Part model, mm, in its own coordinate system. A direction names the side the tool comes from. Give positions to 0.01 mm unless a question says otherwise; leave off trailing zeros. Loops run counter-clockwise (first coordinate to the right, second up) from the corner with the lowest first, then second, coordinate; pieces in that order, holes last. Notation, with made-up numbers: (21, -25) -> (75, -25) arc R8 ccw to (75, -16) -> close; hole circle Ø6 at (-8.5, 49.25). An arc over 180 degrees is marked (long way). Write item = value, one per line.
from build123d import *

# Parameters (mm, degrees)
SKETCH_1_W          = 12.5
SKETCH_1_H          = 12.5
EXTRUDE_1_DEPTH     = 44.8
SKETCH_2_W          = 10
SKETCH_2_H          = 10
CUT_EXTRUDE_1_DEPTH = 44
FILLET_1_R          = 1


with BuildPart() as part:
    # Эскиз1 → Бобышка-Вытянуть1 (new body)
    with BuildSketch(Plane(origin=(0, 0, 0), x_dir=(1, 0, 0), z_dir=(0, 1, 0))):
        with Locations((6.25, 6.25)):
            Rectangle(SKETCH_1_W, SKETCH_1_H)
    extrude(amount=EXTRUDE_1_DEPTH)

    # Эскиз2 → Вырез-Вытянуть1 (cut)
    with BuildSketch(Plane(origin=(0, 44.8, 0), x_dir=(1, 0, 0), z_dir=(0, 1, 0))):
        with Locations((6.25, 6.25)):
            Rectangle(SKETCH_2_W, SKETCH_2_H)
    extrude(amount=-CUT_EXTRUDE_1_DEPTH, mode=Mode.SUBTRACT)

    # Скругление1
    fillet_1_edges = [part.edges().sort_by_distance(p)[0] for p in [
        (6.25, 0, -12.5),
        (6.25, 0, 0),
    ]]
    fillet(fillet_1_edges, radius=FILLET_1_R)


solid = part.part
1) Slice it at B-B, the plane x = 4.75. List the corners of the cut face in (y, z), and give its area (3 significant figures).
Resolved:
outline = (0, -11.5) arc R1 ccw to (1, -12.5) -> (44.8, -12.5) -> (44.8, -11.25) -> (0.8, -11.25) -> (0.8, -1.25) -> (44.8, -1.25) -> (44.8, 0) -> (1, 0) arc R1 ccw to (0, -1) -> close
area = 120 mm²
2) Drill centre lines: line 1 along Z through (x, y) = (11, 18.5); line 2 along X through (y, z) = (7, -8.5); line 3 along Y through (x, z) = (4.75, -10). Where is each one in solid material? Low to high. Write a range as [from, to].
Resolved:
line_1 = [-12.5, -11.25], [-1.25, 0]
line_2 = [0, 1.25], [11.25, 12.5]
line_3 = [0, 0.8]
3) Slice it at C-C, the plane y = 19.5. List the corners of the cut face in (x, z).
Resolved:
outline = (0, -12.5) -> (12.5, -12.5) -> (12.5, 0) -> (0, 0) -> close; hole (1.25, -11.25) -> (11.25, -11.25) -> (11.25, -1.25) -> (1.25, -1.25) -> close
4) Drop flat-ended pins along their axis: P1, Ø6, axis at x = 5, z = -8, coming from the +Y side; P2, Ø6, axis at y = 14, z = -5, coming from the -X side. Give the stop position or say it passes through.
Resolved:
P1 = 0.8
P2 = 0
5) Pull direction Z, two halves, no side cores. Call faces 3 (the face through (12.5, 22, -6)), 4 (the face through (6, 23, 0)), 5 (the face through (6, 23, -1.25)), 6 (the face through (6, 0.8, -6)): pulls with the +Z half, pulls with the -Z half, needs draft (parallel to the pull), parting line crosses it, or undercut.
Resolved:
face_3 = needs draft
face_4 = pulls with the +Z half
face_5 = undercut
face_6 = undercut
6) Which spindle directions (+Z, -Z, +X, -X, +Y, -Y) get a long thin tool onto all of the face, cutting with end or side? Do faces 1 (the face through (1.25, 23, -6)), 2 (the face through (0, 22, -6)). Say none if no direction does.
Resolved:
face_1 = +Y
face_2 = +Z, -Z, -X, +Y, -Y
7) Slice it at A-A, the plane z = -2.5. List the corners of the cut face in (x, y), and give its area (3 significant figures).
Resolved:
outline = (0, 0) -> (12.5, 0) -> (12.5, 44.8) -> (11.25, 44.8) -> (11.25, 0.8) -> (1.25, 0.8) -> (1.25, 44.8) -> (0, 44.8) -> close
area = 120 mm²
